Input: part model. Units: mm. Frame: model coordinates. Face numbers are marked on the shaded views. A direction names the side the tool comes from. Round coordinates to 2 decimals unless told otherwise and drop trailing zeros. Order: outer loops, then holes, each group sorted by start corner. A loop starts at its lowest first (then second) coordinate and runs counter-clockwise, first axis right, second up. Notation, with made-up numbers: (74, 79) - (115, 79) arc R19 ccw to (115, 102) - close; hole circle Ø3 at (-29.5, 3). An arc over 180 degrees is marked (long way). One line per item, written item: value. Start each with the question number.
from build123d import *

# Parameters (mm, degrees)
F1_DEPTH = 10
F2_W     = 34
F2_H     = 15
F3_DEPTH = 5
F4_R     = 2.25
F5_DEPTH = 25
F6_SIZE  = 0.5


with BuildPart() as f1:
    # F0 (on Right) → F1 (new body)
    with BuildSketch(Plane.YZ):
        Polygon((0, 7.5), (-50, 7.5), (-50, 3.25), (-50, 0), (-50, -3.25), (-50, -7.5), (0, -7.5), (0, 0), align=None)
        with BuildLine():
            ThreePointArc((-36.75, -3.25), (-40, 0), (-36.75, 3.25))
            Line((-36.75, 3.25), (-13.25, 3.25))
            ThreePointArc((-13.25, 3.25), (-10, 0), (-13.25, -3.25))
            Line((-13.25, -3.25), (-36.75, -3.25))
        make_face(mode=Mode.SUBTRACT)
    extrude(amount=F1_DEPTH)

    # F2 (on face) → F3 (cut)
    with BuildSketch(Plane.YZ.offset(10)):
        with Locations((-25, 0)):
            Rectangle(F2_W, F2_H)
    extrude(amount=-F3_DEPTH, mode=Mode.SUBTRACT)

    # F4 (on face) → F5 (cut)
    with BuildSketch(Plane.XY.offset(7.5)):
        with Locations((5, -46)):
            Circle(F4_R)
        with Locations((5, -4)):
            Circle(F4_R)
    extrude(amount=-F5_DEPTH, mode=Mode.SUBTRACT)

    # F6
    f6_edges = [f1.edges().sort_by_distance(p)[0] for p in [
        (2.75, -46, 7.5),
        (7.25, -46, 0),
        (2.75, -46, -7.5),
        (2.75, -4, 7.5),
        (7.25, -4, 0),
        (2.75, -4, -7.5),
    ]]
    chamfer(f6_edges, length=F6_SIZE)


solid = f1.part
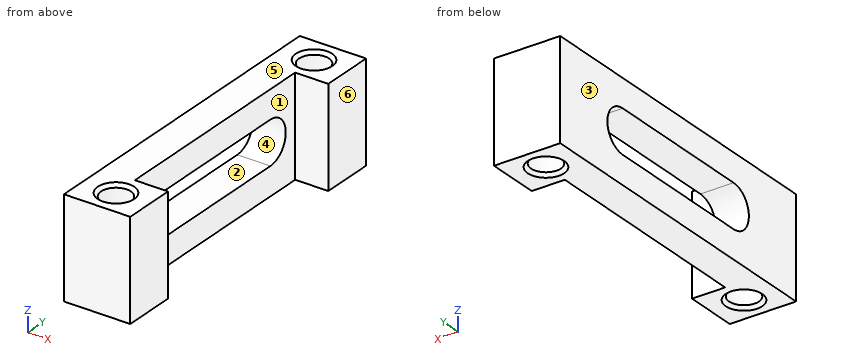
Item 1: Line query: L1, parallel to Y at x = 1.25, z = 0; L2, parallel to Z at x = 1, y = -14; L3, parallel to Y at x = 8.5, z = 0.25. Output: solid intervals per line, ascending.
Item 2: Section query D-D on x = 1.25. Return loops of the section in (y, z).
Item 3: Pull-direction query (Z, two-part tool) for the marked faces 4, 5 and 6; classes: released by +Z, released by -Z, zero draft, split by the parting line, or undercut.
Item 4: Section query B-B on x = 8.5. Return loops of the section in (y, z), and give its area (3 significant figures).
Item 5: Section query A-A on y = -12. Return loops of the section in (x, z).
Item 6: Reachability of the marked faces 1, 2 and 3 from +Z, -Z, +X, -X, +Y, -Y: full face, straight path, thin tool, end or side. Return the list, or none.
Item 7: Section query C-C on z = -5.25. Return loops of the section in (x, y).
Item 8: First-contact query: pin 1 Ø1 at (x, z) = (5, -4.5) entering from +Y. Flat tip, straight axial feed; report the tip coordinate or a pass-through.
Geometry results:
1. L1: y = -50 to -40, -10 to 0
1. L2: z = -7.5 to -3.25, 3.25 to 7.5
1. L3: y = -50 to -42, -8 to 0
2. outline: (-50, -7.5) - (0, -7.5) - (0, 7.5) - (-50, 7.5) - close; hole (-36.75, -3.25) - (-13.25, -3.25) arc R3.25 ccw to (-13.25, 3.25) - (-36.75, 3.25) arc R3.25 ccw to start
3. face 4: undercut
3. face 5: released by +Z
3. face 6: zero draft
4. outline: (-50, -7.5) - (-42, -7.5) - (-42, 7.5) - (-50, 7.5) - close; (-8, -7.5) - (0, -7.5) - (0, 7.5) - (-8, 7.5) - close
4. area: 240 mm^2
5. outline: (0, -7.5) - (5, -7.5) - (5, -3) - (0, -3) - close; (0, 3) - (5, 3) - (5, 7.5) - (0, 7.5) - close
6. face 1: +Z, -Z, +X
6. face 2: +X, -X
6. face 3: +Z, -Z, -X, +Y, -Y
7. outline: (0, -50) - (10, -50) - (10, -42) - (5, -42) - (5, -8) - (10, -8) - (10, 0) - (0, 0) - close; hole circle Ø4.5 at (5, -46); hole circle Ø4.5 at (5, -4)
8. pin 1: stops at y = 0
